Source: CAD feature listing. Evaluate the final solid. Frame: model axes, mm. Round coordinates to 2 decimals unless told otherwise and drop trailing zeros. Loops run counter-clockwise (first coordinate to the right, second up) from the corner with the lowest first, then second, coordinate; pieces in that order, holes last. Notation, with made-up numbers: M 26,80 L 57,80 A15 ccw 57,108 Z; hole C -10.75,-0.75 d7. An arc over 180 degrees is marked long. One line per item, written item: value.
from build123d import *

# Parameters (mm, degrees)
SKETCH1_R                = 59
EXTRUDE1_DEPTH           = 3
EXTRUDE2_DEPTH           = 3
CIRPATTERN1_COUNT        = 6
F_2_0_2_DIAMETER_HOLE1_D = 2
F_2_0_2_DIAMETER_HOLE3_D = 2


with BuildPart() as part:
    # Sketch1 → Extrude1 (new, symmetric)
    with BuildSketch(Plane(origin=(0, 0, 0), x_dir=(0, 0, -1), z_dir=(1, 0, 0))):
        Circle(SKETCH1_R)
        Polygon((14.462624243, 25.05), (-14.462624243, 25.05), (-28.925248486, 0), (-14.462624243, -25.05), (14.462624243, -25.05), (28.925248486, 0), align=None, mode=Mode.SUBTRACT)
    extrude(amount=EXTRUDE1_DEPTH, both=True)

    # Sketch2 → Extrude2 (add, symmetric)
    with BuildSketch(Plane(origin=(0, 0, 0), x_dir=(0, 0, -1), z_dir=(1, 0, 0))):
        with BuildLine():
            Line((-2, 67.961805723), (-0.262709442, 61.478149092))
            ThreePointArc((-0.262709442, 61.478149092), (-0.58620663, 59.77173183), (-2.122608272, 58.961805723))
            ThreePointArc((-2.122608272, 58.961805723), (28.679663449, 51.560419941), (51.21368579, 29.294340542))
            ThreePointArc((51.21368579, 29.294340542), (36.791707484, 48.186627241), (17.927108603, 62.644803614))
            ThreePointArc((17.927108603, 62.644803614), (8.312130826, 66.609702921), (-2, 67.961805723))
        make_face()
    extrude2 = extrude(amount=EXTRUDE2_DEPTH, both=True)

    # CirPattern1: Extrude2 ×6 about axis
    cirpattern1_axis = Axis((0, 0, 0), (1, 0, 0))
    for i in range(1, CIRPATTERN1_COUNT):
        add(extrude2.rotate(cirpattern1_axis, i * 360 / CIRPATTERN1_COUNT))

    # Ø2.0 (2) Diameter Hole1 (through all)
    with Locations(Plane(origin=(3, 0, 0), x_dir=(0, 0, -1), z_dir=(1, 0, 0))):
        with Locations((-14.462624243, 25.05), (14.462624243, 25.05), (28.925248486, 0), (14.462624243, -25.05), (-14.462624243, -25.05), (-28.925248486, 0)):
            Hole(F_2_0_2_DIAMETER_HOLE1_D / 2)

    # Ø2.0 (2) Diameter Hole3 (through all)
    with Locations(Plane(origin=(3, 0, 0), x_dir=(0, 0, -1), z_dir=(1, 0, 0))):
        with Locations((-4.487541414, 25.05)):
            Hole(F_2_0_2_DIAMETER_HOLE3_D / 2)


solid = part.part
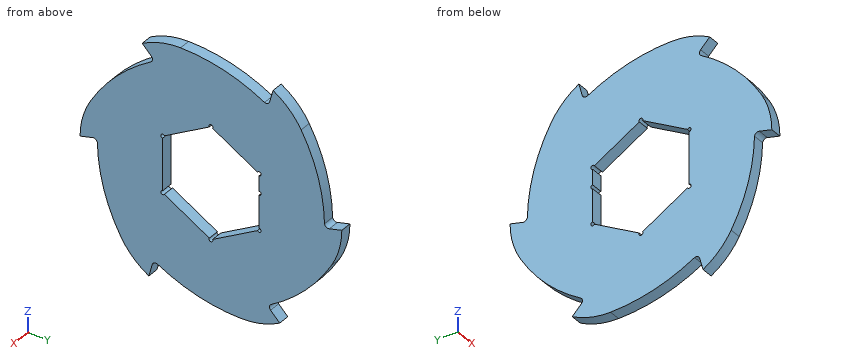
1. Ray query, line 1 (Y direction, x = -1.7, z = -6); line 2 (Z direction, x = -0.8, y = 0.5); line 3 (Y direction, x = -1.85, z = -18.5). Return the intervals inside material, ascending. Write a range as [from, to].
Report:
line 1: y = [-58.81, -25.05], [25.05, 67.15]
line 2: z = [-61.94, -29.79], [29.79, 61.76]
line 3: y = [-57.1, -18.06], [18.06, 62.31]
2. Pin query (flat end, axial travel): pin 1 (1 mm diameter, centred on x = 0.5, z = 12.5, fed in from +Y); pin 2 (2.5 mm diameter, centred on y = -25.05, z = -14.46, fed in from +X); pin 3 (1.6 mm diameter, centred on y = 25.05, z = -14.46, fed in from +X); pin 4 (1 mm diameter, centred on x = 2, z = 35.5, fed in from -Y). Return the tip coordinate at first contact, or that it passes through.
Report:
pin 1: stops at y = 58.21
pin 2: stops at x = 3
pin 3: passes through
pin 4: stops at y = -49.93
3. Section query C-C (z = 32). Return the cut outline in (x, y), and give its area (3 significant figures).
Report:
outline: M -3,-52.65 L 3,-52.65 L 3,53.17 L -3,53.17 Z
area: 635 mm2
4. Section query A-A (y = 4.5). Return the cut outline in (x, z).
Report:
outline: M -3,-62.53 L 3,-62.53 L 3,-26.33 L -3,-26.33 Z; M -3,26.33 L 3,26.33 L 3,60.94 L -3,60.94 Z
5. Section query D-D (z = -36). Return the cut outline in (x, y), and give its area (3 significant figures).
Report:
outline: M -3,-51.54 L 3,-51.54 L 3,48.97 L -3,48.97 Z
area: 603 mm2
6. Section query B-B (z = -5.5). Return the cut outline in (x, y), and give its area (3 significant figures).
Report:
outline: M -3,-58.84 L 3,-58.84 L 3,-25.05 L -3,-25.05 Z; M -3,25.05 L 3,25.05 L 3,67.25 L -3,67.25 Z
area: 456 mm2
